from build123d import *

# Parameters (mm, degrees)
F1_DEPTH = 25
F3_DEPTH = 50
F5_DEPTH = 50
F7_DEPTH = 25.001
F8_R     = 2.75
F9_DEPTH = 10


with BuildPart() as f1:
    # F0 (on Front) → F1 (new body)
    with BuildSketch(Plane.XZ):
        with BuildLine():
            Line((25.636266364, 0), (21, 0))
            ThreePointArc((21, 0), (0, -21), (-21, 0))
            Line((-21, 0), (-25.636266364, 0))
            Line((-25.636266364, 0), (-75, -70.4987177976))
            Line((-75, -70.4987177976), (-17.6593568998, -110.6490683422))
            Line((-17.6593568998, -110.6490683422), (-15, -106.8511130866))
            Line((-15, -106.8511130866), (15, -106.8511130866))
            Line((15, -106.8511130866), (17.6593568998, -110.6490683422))
            Line((17.6593568998, -110.6490683422), (75, -70.4987177976))
            Line((75, -70.4987177976), (25.636266364, 0))
        make_face()
    extrude(amount=F1_DEPTH)

    # F2 (on face) → F3 (cut)
    with BuildSketch(Plane(origin=(-57.7978070699, 0, -82.543822961), x_dir=(0.8191520443, 0, -0.5735764364), z_dir=(-0.5735764364, 0, -0.8191520443))):
        with BuildLine():
            ThreePointArc((34, 0), (14, 20), (-6, 0))
            Line((-6, 0), (34, 0))
        make_face()
    extrude(amount=-F3_DEPTH, mode=Mode.SUBTRACT)

    # F4 (on face) → F5 (cut)
    with BuildSketch(Plane(origin=(57.7978070699, 0, -82.543822961), x_dir=(0.8191520443, 0, 0.5735764364), z_dir=(0.5735764364, 0, -0.8191520443))):
        with BuildLine():
            ThreePointArc((6, 0), (-14, 20), (-34, 0))
            Line((-34, 0), (6, 0))
        make_face()
    extrude(amount=-F5_DEPTH, mode=Mode.SUBTRACT)

    # F6 (on face) → F7 (cut, through all)
    with BuildSketch(Plane(origin=(0, 0, 0), x_dir=(-1, 0, 0), z_dir=(0, 1, 0))):
        with BuildLine():
            ThreePointArc((-61.5432601044, -64.3563525056), (-65.5598750956, -67.8788293138), (-60.3705953043, -66.6090206274))
            ThreePointArc((-60.3705953043, -66.6090206274), (-60.6813155131, -65.339211941), (-61.5432601044, -64.3563525056))
        make_face()
        with BuildLine():
            ThreePointArc((36.0191086867, -27.9040865347), (36.881053278, -26.9212270993), (37.1917734868, -25.6514184129))
            ThreePointArc((37.1917734868, -25.6514184129), (32.0024936955, -24.3816097265), (36.0191086867, -27.9040865347))
        make_face()
        with BuildLine():
            ThreePointArc((65.8705953043, -66.6090206274), (64.3904039907, -64.1697408361), (61.5432601044, -64.3563525056))
            ThreePointArc((61.5432601044, -64.3563525056), (61.8507866179, -69.0483004186), (65.8705953043, -66.6090206274))
        make_face()
        with BuildLine():
            ThreePointArc((0, -49.6011130866), (1.9445436483, -48.7956567348), (2.75, -46.8511130866))
            ThreePointArc((2.75, -46.8511130866), (-1.9445436483, -44.9065694383), (0, -49.6011130866))
        make_face()
        with BuildLine():
            ThreePointArc((2.75, -91.8511130866), (1.9445436483, -89.9065694383), (0, -89.1011130866))
            ThreePointArc((0, -89.1011130866), (-1.9445436483, -93.7956567348), (2.75, -91.8511130866))
        make_face()
        with BuildLine():
            ThreePointArc((-31.6917734868, -25.6514184129), (-35.7115821732, -23.2121386217), (-36.0191086867, -27.9040865347))
            ThreePointArc((-36.0191086867, -27.9040865347), (-33.1719648004, -28.0906982041), (-31.6917734868, -25.6514184129))
        make_face()
    extrude(amount=-F7_DEPTH, mode=Mode.SUBTRACT)

    # F8 (on face) → F9 (cut)
    with BuildSketch(Plane.XZ.offset(25)):
        Polygon((-30.1917734868, -28.105157057), (-30.1917734868, -23.1976797689), (-34.4417734868, -20.7439411248), (-38.6917734868, -23.1976797689), (-38.6917734868, -28.105157057), (-34.4417734868, -30.558895701), align=None)
        with Locations((-34.4417734868, -25.6514184129)):
            Circle(F8_R, mode=Mode.SUBTRACT)
        Polygon((-58.8705953043, -69.0627592714), (-58.8705953043, -64.1552819833), (-63.1205953043, -61.7015433392), (-67.3705953043, -64.1552819833), (-67.3705953043, -69.0627592714), (-63.1205953043, -71.5164979155), align=None)
        with Locations((-63.1205953043, -66.6090206274)):
            Circle(F8_R, mode=Mode.SUBTRACT)
        Polygon((4.25, -94.3048517306), (4.25, -89.3973744425), (0, -86.9436357985), (-4.25, -89.3973744425), (-4.25, -94.3048517306), (0, -96.7585903747), align=None)
        with Locations((0, -91.8511130866)):
            Circle(F8_R, mode=Mode.SUBTRACT)
        Polygon((4.25, -49.3048517306), (4.25, -44.3973744425), (0, -41.9436357985), (-4.25, -44.3973744425), (-4.25, -49.3048517306), (0, -51.7585903747), align=None)
        with Locations((0, -46.8511130866)):
            Circle(F8_R, mode=Mode.SUBTRACT)
        Polygon((30.1917734868, -23.1976797689), (30.1917734868, -28.105157057), (34.4417734868, -30.558895701), (38.6917734868, -28.105157057), (38.6917734868, -23.1976797689), (34.4417734868, -20.7439411248), align=None)
        with Locations((34.4417734868, -25.6514184129)):
            Circle(F8_R, mode=Mode.SUBTRACT)
        Polygon((58.8705953043, -64.1552819833), (58.8705953043, -69.0627592714), (63.1205953043, -71.5164979155), (67.3705953043, -69.0627592714), (67.3705953043, -64.1552819833), (63.1205953043, -61.7015433392), align=None)
        with Locations((63.1205953043, -66.6090206274)):
            Circle(F8_R, mode=Mode.SUBTRACT)
    extrude(amount=-F9_DEPTH, mode=Mode.SUBTRACT)


solid = f1.part
Here's how the part is built. I have some questions about the finished solid (model axes, mm). A direction names the side the tool comes from. Coordinates: 2 decimals unless noted, no trailing zeros. Order: outer loops, then holes, each group sorted by start corner. A loop starts at its lowest first (then second) coordinate and runs counter-clockwise, first axis right, second up. Notation, with made-up numbers: (89, -22) - (106, -22) arc R23 ccw to (106, 5) - close; hole circle Ø9 at (59.5, -32). An arc over 180 degrees is marked (long way). Use CSV: the item, a comma, the result in double quotes. Start each with the question number.
1. I'm going to push flat-ended pins straight in: pin 1 (4 mm diameter, centred on y = -21, z = -66.5, fed in from -X); pin 2 (1.5 mm diameter, centred on x = -46, z = -92.5, fed in from +Y); pin 3 (4 mm diameter, centred on y = -21.5, z = -91, fed in from +X); pin 4 (5.5 mm diameter, centred on y = -18.5, z = -91, fed in from -X). Where does each tip first touch, or does it pass through?
2. Please list where these lines run through material, in increasing order: line 1 (X direction, y = -2.75, z = -48); line 2 (X direction, y = -1.25, z = -69); line 3 (Z direction, x = -36.5, y = -6.5). Write a range as from..to.
3. If we mould it in two halves opening along Z, with no side actions, what happens to faces 1 (the face through (16.31, -12.32, -108.72)), 2 (the face through (4.25, -20, -47)), 3 (the face through (-23, -12, 0))? For each: +Z half, -Z half, draft (parallel to the pull), parting line (faces both ways), or undercut.
4. Suppose I cut it at B-B on y = -23. Give the number of separate pieces and of enclosed holes in the cut face, then the cut area to 3 significant figures.
5. Suppose I cut it at A-A on y = -6.75. List the corners of the cut face in (x, z) for me.
6. For faces 4 (the face through (30.192, -20, -26)), 5 (the face through (17.42, -7.92, -49.78)), 6 (the face through (23, -12, 0)), which set-ups out of +Z, -Z, +X, -X, +Y, -Y let a thin tool reach every point of the face, with its end or its side?
Output:
1,pin 1,"stops at x = -73.6"
1,pin 2,"passes through"
1,pin 3,"stops at x = 48.58"
1,pin 4,"stops at x = -49.27"
2,line 1,"x = -59.25..-40.7, -19.96..-2.5, 2.5..19.96, 40.7..59.25"
2,line 2,"x = -73.95..-64.48, -61.76..-55.59, -6.86..6.86, 55.59..61.76, 64.48..73.95"
2,line 3,"z = -43.56..-27.48, -23.83..-15.52"
3,face 1,"-Z half"
3,face 2,"undercut"
3,face 3,"+Z half"
4,separate pieces,"1"
4,enclosed holes,"6"
4,area,"9,620 mm2"
5,outline,"(-75, -70.5) - (-61.75, -79.78) - (-33.07, -38.82) - (-2.23, -60.41) - (-30.91, -101.37) - (-17.66, -110.65) - (-15, -106.85) - (15, -106.85) - (17.66, -110.65) - (30.91, -101.37) - (2.23, -60.41) - (33.07, -38.82) - (61.75, -79.78) - (75, -70.5) - (25.64, 0) - (21, 0) arc R21 cw to (-21, 0) - (-25.64, 0) - close; hole circle Ø5.5 at (-63.12, -66.61); hole circle Ø5.5 at (-34.44, -25.65); hole circle Ø5.5 at (0, -91.85); hole circle Ø5.5 at (0, -46.85); hole circle Ø5.5 at (34.44, -25.65); hole circle Ø5.5 at (63.12, -66.61)"
6,face 4,"-Y"
6,face 5,"+Y"
6,face 6,"+Z, +X, -X, +Y, -Y"
